The model under review builds one solid part; all positions refer to its coordinate system, in mm. A direction names the side the tool comes from. Round coordinates to 2 decimals unless told otherwise and drop trailing zeros. Order: outer loops, then holes, each group sorted by start corner. A loop starts at its lowest first (then second) coordinate and runs counter-clockwise, first axis right, second up. Notation, with made-up numbers: (7.5, -14) -> (48.5, -14) arc R19 cw to (48.5, -2) -> close; hole circle Ø11 at (81.5, 55.25). An arc over 180 degrees is marked (long way). Use a Markdown table: item, result. Add a question column.
```python
from build123d import *

# Parameters (mm, degrees)
BOSS_EXTRUDE1_DEPTH = 30
CUT_EXTRUDE2_START  = -10
SKETCH2_R           = 9.068137576
SKETCH2_R_2         = 5.1145
CUT_EXTRUDE2_DEPTH  = 10


with BuildPart() as part:
    # Sketch1 → Boss-Extrude1 (new body)
    with BuildSketch(Plane.XY):
        with BuildLine():
            Line((-2, 7), (2, 7))
            Line((2, 7), (2, 4.707240195))
            ThreePointArc((2, 4.707240195), (0, -5.1145), (-2, 4.707240195))
            Line((-2, 4.707240195), (-2, 7))
        make_face()
    extrude(amount=BOSS_EXTRUDE1_DEPTH)

    # Sketch2 → Cut-Extrude2 (cut)
    with BuildSketch(Plane.XY.offset(30).offset(CUT_EXTRUDE2_START)):
        Circle(SKETCH2_R)
        Circle(SKETCH2_R_2, mode=Mode.SUBTRACT)
    extrude(amount=-CUT_EXTRUDE2_DEPTH, mode=Mode.SUBTRACT)


solid = part.part
```
Q1. Add section B-B (x = 0). Write out the cut boundary in (y, z).
Q2. Machinability: for faces 4 (the flat face through (0, 7, 25)), 5 (the flat face through (2, 6, 25)), 6 (the flat face through (-2, 6, 25)), which of the approach directions +Z, -Z, +X, -X, +Y, -Y give a long, thin tool a straight path to every point of the face, cutting with its end or side? Answer none if there is none.
Q3. Add section C-C (z = 20.5). Write out the cut boundary in (x, y).
Q4. Add section A-A (y = 5.75). Write out the cut boundary in (x, z).
Q5. Wall thickness on line 1 (Z direction, x = 1.5, y = 6.75); line 2 (X direction, y = 5.25, z = 8.5); line 3 (X direction, y = -3.75, z = 26): over which ranges is each line inside the solid? List them lowest first. Write a range as [from, to].
Q6. Insertion check: pin 1 (1.5 mm diameter, centred on y = 5.5, z = 19.5, fed in from +X); pin 2 (0.7 mm diameter, centred on y = 6.5, z = 23.5, fed in from -X); pin 3 (1 mm diameter, centred on y = 1, z = 21, fed in from +X). Each pin has a flat end and moves straight along its axis. Give the tip position at first contact, or say it passes through.
Q7. Mouldability with a two-part tool opening along Z and no side actions: class faces 1 (the flat face through (0, 1, 0)), 2 (the flat face through (0, 6, 20)), 3 (the flat face through (-2, 6, 5)) as pulls with the +Z half, pulls with the -Z half, needs draft (parallel to the pull), parting line crosses it, or undercut.
Q8. Add section D-D (y = 1.25). Write out the cut boundary in (x, z), then the cut area to 3 significant figures.
Report:
| question | item | result |
|---|---|---|
| 1 | outline | (-5.11, 0) -> (7, 0) -> (7, 10) -> (5.11, 10) -> (5.11, 20) -> (7, 20) -> (7, 30) -> (-5.11, 30) -> close |
| 2 | face 4 | +Z, -Z, +X, -X, +Y |
| 2 | face 5 | +Z, -Z, +X, +Y |
| 2 | face 6 | +Z, -Z, -X, +Y |
| 3 | outline | (-2, 4.71) arc R5.11 ccw (long way) to (2, 4.71) -> (2, 7) -> (-2, 7) -> close |
| 4 | outline | (-2, 0) -> (2, 0) -> (2, 10) -> (-2, 10) -> close; (-2, 20) -> (2, 20) -> (2, 30) -> (-2, 30) -> close |
| 5 | line 1 | z = [0, 10], [20, 30] |
| 5 | line 2 | x = [-2, 2] |
| 5 | line 3 | x = [-3.48, 3.48] |
| 6 | pin 1 | stops at x = 2 |
| 6 | pin 2 | stops at x = -2 |
| 6 | pin 3 | stops at x = 5.09 |
| 7 | face 1 | pulls with the -Z half |
| 7 | face 2 | undercut |
| 7 | face 3 | needs draft |
| 8 | outline | (-4.96, 0) -> (4.96, 0) -> (4.96, 30) -> (-4.96, 30) -> close |
| 8 | area | 298 mm² |
